Check sheet for the modelled part. Datum: model origin and axes. Units: mm. A direction names the side the tool comes from. Give positions to 0.01 mm unless a question says otherwise; leave off trailing zeros. Order: outer loops, then holes, each group sorted by start corner. A loop starts at its lowest first (then second) coordinate and runs counter-clockwise, first axis right, second up. Notation, with made-up numbers: (5, 83.25) -> (58, 83.25) arc R11 cw to (58, 94.25) -> close; hole circle Ø1 at (-10, 76). An arc over 180 degrees is marked (long way). One line per question, with ' | ' between items. Start each with the question number.
from build123d import *

# Parameters (mm, degrees)
SKETCH_1_R      = 10
SKETCH_1_R_2    = 7.6
EXTRUDE_1_DEPTH = 2
EXTRUDE_START   = -2
EXTRUDE_2_DEPTH = 2


with BuildPart() as part:
    # ｽｹｯﾁ1 → ﾎﾞｽ - 押し出し1 (new body)
    with BuildSketch(Plane.XY):
        Circle(SKETCH_1_R)
        Circle(SKETCH_1_R_2, mode=Mode.SUBTRACT)
    extrude(amount=EXTRUDE_1_DEPTH)

    # ｽｹｯﾁ2 → ﾎﾞｽ - 押し出し2 (add)
    with BuildSketch(Plane.XY.offset(2).offset(EXTRUDE_START)):
        with BuildLine():
            Line((0, 30), (0, 10))
            ThreePointArc((0, 10), (3.826834324, 9.238795325), (7.071067812, 7.071067812))
            Line((7.071067812, 7.071067812), (21.213203436, 21.213203436))
            ThreePointArc((21.213203436, 21.213203436), (11.480502971, 27.716385975), (0, 30))
        make_face()
        with BuildLine():
            Line((21.213203436, -21.213203436), (7.071067812, -7.071067812))
            ThreePointArc((7.071067812, -7.071067812), (9.238795325, -3.826834324), (10, 0))
            Line((10, 0), (30, 0))
            ThreePointArc((30, 0), (27.716385975, -11.480502971), (21.213203436, -21.213203436))
        make_face()
        with BuildLine():
            Line((-21.213203436, -21.213203436), (-7.071067812, -7.071067812))
            ThreePointArc((-7.071067812, -7.071067812), (-3.826834324, -9.238795325), (0, -10))
            Line((0, -10), (0, -30))
            ThreePointArc((0, -30), (-11.480502971, -27.716385975), (-21.213203436, -21.213203436))
        make_face()
        with BuildLine():
            Line((-21.213203436, 21.213203436), (-7.071067812, 7.071067812))
            ThreePointArc((-7.071067812, 7.071067812), (-9.238795325, 3.826834324), (-10, 0))
            Line((-10, 0), (-30, 0))
            ThreePointArc((-30, 0), (-27.716385975, 11.480502971), (-21.213203436, 21.213203436))
        make_face()
    extrude(amount=EXTRUDE_2_DEPTH)


solid = part.part
1. Cross-section at C-C on y = -9. Record the boundary of the cut face in (x, z), and give its area (3 significant figures).
2. Cross-section at A-A on z = 1.65. Record the boundary of the cut face in (x, y).
3. Tool access check on faces 5 (the face through (-14, 14, 1)), 6 (the face through (9.26, 3.78, 0.99)), 7 (the face through (-9.26, -3.78, 0.99)). Record the directions out of +Z, -Z, +X, -X, +Y, -Y that give a thin tool (end or side, any length) a straight path to the whole face; none if there is none.
4. Mould release check, pull along X, two halves, no side actions. Record for faces 1 (the face through (-4, 7, 2)), 2 (the face through (-3.78, 9.26, 0.99)), 3 (the face through (14, 14, 1)), 4 (the face through (-27.78, 11.33, 0.99)): +X half, -X half, draft (parallel to the pull), parting line (faces both ways), or undercut.
5. Cross-section at B-B on x = 2. Record the boundary of the cut face in (y, z).
6. Scan lines: probe 1 along X at (y, z) = (-19, 1.35); probe 2 along Y at (x, z) = (-1.5, 1.35); probe 3 along X at (y, z) = (7, 1.4). Record each from-to range of solid material in increasing order.
7. Go/stop test with flat-tipped pins: pin 1 (1 mm diameter, centred on y = -24, z = 1, fed in from +X); pin 2 (0.6 mm diameter, centred on x = -18, z = 1.5, fed in from -Y); pin 3 (0.6 mm diameter, centred on y = 25, z = 1, fed in from -X). Record where each tip stops, or that it passes through.
Response values:
1) outline: (-9, 0) -> (4.36, 0) -> (4.36, 2) -> (-9, 2) -> close; (9, 0) -> (28.62, 0) -> (28.62, 2) -> (9, 2) -> close | area: 66.0 mm²
2) outline: (-30, 0) -> (-10, 0) arc R10 ccw to (-7.07, -7.07) -> (-21.21, -21.21) arc R30 ccw to (0, -30) -> (0, -10) arc R10 ccw to (7.07, -7.07) -> (21.21, -21.21) arc R30 ccw to (30, 0) -> (10, 0) arc R10 ccw to (7.07, 7.07) -> (21.21, 21.21) arc R30 ccw to (0, 30) -> (0, 10) arc R10 ccw to (-7.07, 7.07) -> (-21.21, 21.21) arc R30 ccw to start; hole circle Ø15.2 at (0, 0)
3) face 5: +Z, -Z, +Y | face 6: +Z, -Z, +X | face 7: +Z, -Z, -X
4) face 1: draft | face 2: undercut | face 3: +X half | face 4: -X half
5) outline: (-9.8, 0) -> (-7.33, 0) -> (-7.33, 2) -> (-9.8, 2) -> close; (7.33, 0) -> (29.93, 0) -> (29.93, 2) -> (7.33, 2) -> close
6) probe 1: x = -19 to 0, 19 to 23.22 | probe 2: y = -29.96 to -7.45, 7.45 to 9.89 | probe 3: x = -29.17 to -2.96, 2.96 to 7.14
7) pin 1: stops at x = 0 | pin 2: stops at y = -24.22 | pin 3: stops at x = 0
